The model under review builds one solid part; all positions refer to its coordinate system, in mm. A direction names the side the tool comes from. Round coordinates to 2 decimals unless told otherwise and drop trailing zeros. Write each loop counter-clockwise with the first axis right and the second up, starting at its lowest first coordinate (ties: lowest second). Pieces come first, ordered by that corner, then holes. Notation, with made-up numbers: M 63.25,-15.75 L 111.25,-15.75 A17 cw 111.25,-7.75 Z; hole C 75,19 d11. An arc over 180 degrees is marked long. One line per item, written item: value. Start each with the question number.
1) Take a section at A-A, the plane x = 10. Write out the cut boundary in (y, z), and give its area (3 significant figures).
2) Wall thickness on probe 1 along Y at (x, z) = (10, 8.75); probe 2 along X at (y, z) = (39, 16.5); probe 3 along X at (y, z) = (34.5, 12.25): over which ranges is each line inside the solid? List them lowest first.
3) Take a section at B-B, the plane y = 34.5. Write out the cut boundary in (x, z), and give its area (3 significant figures).
4) Tool access review of faces 4 (the face through (19, 31, 16)), 5 (the face through (0, 40.5, 16)), 6 (the face through (0.46, 28.84, 4.49)), 7 (the face through (0, 25, 10)): name each direction out of +Z, -Z, +X, -X, +Y, -Y from which nothing blocks a thin tool from reaching the whole face with its end or side.
5) For P1, Ø0.9, axis at y = 32, z = 17, coming from the +X side; P2, Ø9.5, axis at x = 0.5, y = 22, coming from the +Z side; P3, Ø1.8, axis at x = -10, y = 35.37, coming from the -Z side; P4, Ø6, axis at y = 45, z = 12, coming from the +X side, all flat-tipped, find the tip position at first contact; note any pin that passes through.
6) Mouldability with a two-part tool opening along Z and no side actions: class faces 1 (the face through (0, 48.37, 11)), 2 (the face through (-6, 22, 9)), 3 (the face through (-11, 34, 18)) as +Z half, -Z half, draft (parallel to the pull), parting line (faces both ways), or undercut.
7) Take a section at D-D, the plane z = 8.25. Write out the cut boundary in (x, y).
8) Take a section at C-C, the plane y = 39.5. Write out the cut boundary in (x, z).
from build123d import *

# Parameters (mm, degrees)
CROQUIS3_W                   = 38
CROQUIS3_H                   = 38
SALIENTE_EXTRUIR9_DEPTH      = 1
SALIENTE_EXTRUIR10_START     = -11
SALIENTE_EXTRUIR10_OUTLINE_W = 38
SALIENTE_EXTRUIR10_OUTLINE_H = 38
SALIENTE_EXTRUIR10_DEPTH     = 10
CROQUIS13_W                  = 38
CROQUIS13_H                  = 38
SALIENTE_EXTRUIR15_DEPTH     = 3
CROQUIS14_R                  = 1.5
CORTAR_EXTRUIR1_DEPTH        = 14
CROQUIS15_W                  = 38
CROQUIS15_H                  = 24.129942315
CROQUIS15_R                  = 3.5
SALIENTE_EXTRUIR16_DEPTH     = 1
CORTAR_EXTRUIR2_DEPTH        = 14
SALIENTE_EXTRUIR17_DEPTH     = 5
SALIENTE_EXTRUIR18_DEPTH     = 5
CORTAR_EXTRUIR3_DEPTH        = 3
REDONDEO11_R                 = 1
CROQUIS21_R                  = 1.5
CORTAR_EXTRUIR4_DEPTH        = 11
SALIENTE_EXTRUIR20_START     = 3
CROQUIS22_R                  = 3
CROQUIS22_R_2                = 1.5
SALIENTE_EXTRUIR20_DEPTH     = 3


# Read off the part's stored shape, not the designer's step: Saliente-Extruir10
with BuildPart() as part:
    # Croquis3 → Saliente-Extruir9 (new body)
    with BuildSketch(Plane.XY.offset(5)):
        Polygon((19, -5.370057685), (26.870057685, 2.5), (26.870057685, 40.5), (19, 48.370057685), (-19, 48.370057685), (-26.870057685, 40.5), (-26.870057685, 2.5), (-19, -5.370057685), align=None)
        with Locations((0, 21.5)):
            Rectangle(CROQUIS3_W, CROQUIS3_H, mode=Mode.SUBTRACT)
    extrude(amount=-SALIENTE_EXTRUIR9_DEPTH)

    # Saliente-Extruir10 outline → Saliente-Extruir10 (add)
    with BuildSketch(Plane(origin=(0, 0, 4), x_dir=(-1, 0, 0), z_dir=(0, 0, -1)).offset(SALIENTE_EXTRUIR10_START)):
        Polygon((-26.870057685, 2.5), (-19, -5.370057685), (19, -5.370057685), (26.870057685, 2.5), (26.870057685, 40.5), (19, 48.370057685), (-19, 48.370057685), (-26.870057685, 40.5), align=None)
        with Locations((0, 21.5)):
            Rectangle(SALIENTE_EXTRUIR10_OUTLINE_W, SALIENTE_EXTRUIR10_OUTLINE_H, mode=Mode.SUBTRACT)
    extrude(amount=SALIENTE_EXTRUIR10_DEPTH)

    # Croquis13 → Saliente-Extruir15 (add)
    with BuildSketch(Plane.XY.offset(15)):
        with BuildLine():
            Line((-22.5, 44.870057685), (-22.5, -1))
            Line((-22.5, -1), (22.5, -1))
            Line((22.5, -1), (22.5, 44.870057685))
            Line((22.5, 44.870057685), (19.292893219, 48.077164466))
            ThreePointArc((19.292893219, 48.077164466), (18.96846987, 48.293937218), (18.585786438, 48.370057685))
            Line((18.585786438, 48.370057685), (-18.585786438, 48.370057685))
            ThreePointArc((-18.585786438, 48.370057685), (-18.96846987, 48.293937218), (-19.292893219, 48.077164466))
            Line((-19.292893219, 48.077164466), (-22.5, 44.870057685))
        make_face()
        with Locations((0, 21.5)):
            Rectangle(CROQUIS13_W, CROQUIS13_H, mode=Mode.SUBTRACT)
    extrude(amount=SALIENTE_EXTRUIR15_DEPTH)

    # Croquis14 → Cortar-Extruir1 (cut)
    with BuildSketch(Plane(origin=(0, 0, 4), x_dir=(-1, 0, 0), z_dir=(0, 0, -1))):
        with Locations((10, 45.37415474)):
            Circle(CROQUIS14_R)
        with Locations(Location((-10, 45.37415474, 0), (0, 0, 180))):
            Circle(CROQUIS14_R)
    extrude(amount=-CORTAR_EXTRUIR1_DEPTH, mode=Mode.SUBTRACT)

    # Croquis15 → Saliente-Extruir16 (add)
    with BuildSketch(Plane(origin=(0, 0, 4), x_dir=(-1, 0, 0), z_dir=(0, 0, -1))):
        with Locations((0, 28.435028843)):
            Rectangle(CROQUIS15_W, CROQUIS15_H)
        with Locations((0, 25.370057685)):
            Circle(CROQUIS15_R, mode=Mode.SUBTRACT)
    extrude(amount=-SALIENTE_EXTRUIR16_DEPTH)

    # Croquis16 → Cortar-Extruir2 (cut)
    with BuildSketch(Plane(origin=(0, 0, 4), x_dir=(-1, 0, 0), z_dir=(0, 0, -1))):
        Polygon((-19, 2.5), (-19, 16.370057685), (-26.870057685, 24.24011537), (-26.870057685, 2.5), (-19, -5.370057685), (19, -5.370057685), (26.870057685, 2.5), (26.870057685, 24.24011537), (19, 16.370057685), (19, 2.5), align=None)
    extrude(amount=-CORTAR_EXTRUIR2_DEPTH, mode=Mode.SUBTRACT)

    # Croquis17 → Saliente-Extruir17 (add)
    with BuildSketch(Plane.XY.offset(5)):
        Polygon((6, 31.370057685), (6, 25.370057685), (6, 19.370057685), (6, 16.370057685), (19, 16.370057685), (19, 40.5), (-19, 40.5), (-19, 16.370057685), (-6, 16.370057685), (-6, 19.370057685), (-6, 31.370057685), align=None)
    extrude(amount=SALIENTE_EXTRUIR17_DEPTH)

    # Croquis18 → Saliente-Extruir18 (add)
    with BuildSketch(Plane.XY.offset(10)):
        Polygon((-19, 40.5), (-19, 16.370057685), (-6, 16.370057685), (-6, 19.370057685), (6, 19.370057685), (6, 16.370057685), (19, 16.370057685), (19, 40.5), align=None)
    extrude(amount=SALIENTE_EXTRUIR18_DEPTH)

    # Croquis19 → Cortar-Extruir3 (cut)
    with BuildSketch(Plane.XY.offset(18)):
        Polygon((-22.5, 19.870057685), (-19, 16.370057685), (-19, 21.370057685), (-22.5, 21.370057685), align=None)
        Polygon((19, 16.370057685), (22.5, 19.870057685), (22.5, 21.370057685), (19, 21.370057685), align=None)
    extrude(amount=-CORTAR_EXTRUIR3_DEPTH, mode=Mode.SUBTRACT)

    # Redondeo11
    redondeo11_edges = [part.edges().sort_by_distance(p)[0] for p in [
        (26.870057685, 40.5, 10),
        (19, 48.370057685, 10),
        (-19, 48.370057685, 10),
        (-26.870057685, 40.5, 10),
        (26.870057685, 24.24011537, 9.5),
        (19, 16.370057685, 9.5),
        (-26.870057685, 24.24011537, 9.5),
        (-19, 16.370057685, 9.5),
    ]]
    fillet(redondeo11_edges, radius=REDONDEO11_R)

    # Croquis21 → Cortar-Extruir4 (cut)
    with BuildSketch(Plane.XY.offset(15)):
        with Locations((-10, 35.37415474)):
            Circle(CROQUIS21_R)
        with Locations((10, 35.37415474)):
            Circle(CROQUIS21_R)
    extrude(amount=-CORTAR_EXTRUIR4_DEPTH, mode=Mode.SUBTRACT)

    # Croquis22 → Saliente-Extruir20 (add)
    # profile 1 of 2: a face of its own
    with BuildSketch(Plane.XY.offset(15).offset(SALIENTE_EXTRUIR20_START)):
        with Locations(Location((-10, 35.37415474, 0), (0, 0, 180))):
            Circle(CROQUIS22_R)
        with Locations((-10, 35.37415474)):
            Circle(CROQUIS22_R_2, mode=Mode.SUBTRACT)
    # profile 2 of 2: a face of its own
    with BuildSketch(Plane.XY.offset(15).offset(SALIENTE_EXTRUIR20_START)):
        with Locations(Location((10, 35.37415474, 0), (0, 0, 180))):
            Circle(CROQUIS22_R)
        with Locations((10, 35.37415474)):
            Circle(CROQUIS22_R_2, mode=Mode.SUBTRACT)
    extrude(amount=-SALIENTE_EXTRUIR20_DEPTH)

    # Croquis23 → Cortar-Revolución1 (revolve, cut)
    with BuildSketch(Plane.XY.offset(18)):
        Polygon((-1.8, 48.370057685), (-1.8, 44.97415474), (-1.8, 40.5), (0.2, 40.5), (0.2, 48.370057685), align=None)
    revolve(axis=Axis((-1.8, 44.97415474, 18), (0, 1, 0)), mode=Mode.SUBTRACT)


solid = part.part
Checked values:
1. outline: M 16.37,4 L 33.87,4 L 33.87,18 L 32.37,18 L 32.37,15 L 16.37,15 Z; M 36.87,4 L 43.87,4 L 43.87,18 L 40.5,18 L 40.5,15 L 38.37,15 L 38.37,18 L 36.87,18 Z; M 46.87,4 L 48.37,4 L 48.37,18 L 46.87,18 Z
1. area: 310 mm2
2. probe 1: y = 16.37 to 33.87, 36.87 to 43.87, 46.87 to 48.37
2. probe 2: x = -22.5 to -19, 19 to 22.5
2. probe 3: x = -26.87 to -11.22, -8.78 to 8.78, 11.22 to 26.87
3. outline: M -26.87,4 L -11.22,4 L -11.22,18 L -12.87,18 L -12.87,15 L -19,15 L -19,18 L -22.5,18 L -22.5,15 L -26.87,15 Z; M -8.78,4 L 8.78,4 L 8.78,18 L 7.13,18 L 7.13,15 L -7.13,15 L -7.13,18 L -8.78,18 Z; M 11.22,4 L 26.87,4 L 26.87,15 L 22.5,15 L 22.5,18 L 19,18 L 19,15 L 12.87,15 L 12.87,18 L 11.22,18 Z
3. area: 578 mm2
4. face 4: +Z, -Y
4. face 5: +Z
4. face 6: -Z
4. face 7: -Y
5. P1: stops at x = 22.5
5. P2: stops at z = 15
5. P3: passes through
5. P4: stops at x = 25.37
6. face 1: draft
6. face 2: undercut
6. face 3: +Z half
7. outline: M -26.87,24.65 A1 ccw -26.58,23.95 L -19.29,16.66 A1 ccw -18.59,16.37 L -6,16.37 L -6,31.37 L 6,31.37 L 6,16.37 L 18.59,16.37 A1 ccw 19.29,16.66 L 26.58,23.95 A1 ccw 26.87,24.65 L 26.87,40.09 A1 ccw 26.58,40.79 L 19.29,48.08 A1 ccw 18.59,48.37 L -18.59,48.37 A1 ccw -19.29,48.08 L -26.58,40.79 A1 ccw -26.87,40.09 Z; hole C -10,35.37 d3; hole C -10,45.37 d3; hole C 10,35.37 d3; hole C 10,45.37 d3
8. outline: M -26.87,4 L 26.87,4 L 26.87,15 L 22.5,15 L 22.5,18 L 19,18 L 19,15 L -19,15 L -19,18 L -22.5,18 L -22.5,15 L -26.87,15 Z
